Verification items for this drawing (mm, ordinates from the low corner). A direction names the side the tool comes from. Coordinates: 2 decimals unless noted, no trailing zeros. Order: outer loops, then holes, each group sorted by start corner. A loop starts at its lowest first (then second) coordinate and runs counter-clockwise, first axis right, second up.
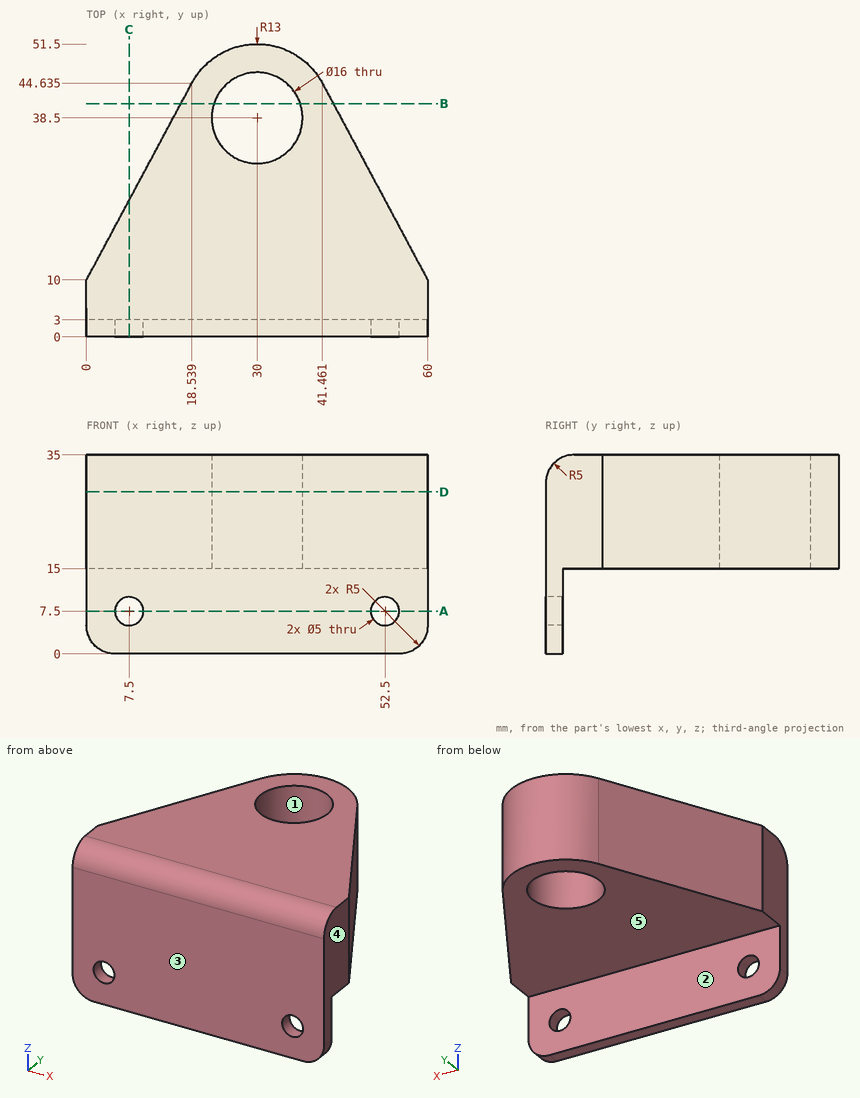
(1) Cross-section at A-A (z = 7.5). Enter the section's corners in (x, y), and give its area (3 significant figures).
Filled in:
outline: (0, 0) - (5, 0) - (5, 3) - (0, 3) - close; (10, 0) - (50, 0) - (50, 3) - (10, 3) - close; (55, 0) - (60, 0) - (60, 3) - (55, 3) - close
area: 150 mm2
(2) Cross-section at B-B (y = 41). Enter the section's corners in (x, z), and give its area (3 significant figures).
Filled in:
outline: (16.59, 15) - (22.4, 15) - (22.4, 35) - (16.59, 35) - close; (37.6, 15) - (43.41, 15) - (43.41, 35) - (37.6, 35) - close
area: 232 mm2
(3) Thickness scan on probe 1 along Y at (x, z) = (30, 22); probe 2 along X at (y, z) = (1, 7); probe 3 along Y at (x, z) = (57, 14). Record the ranges inside material, lowest first.
Filled in:
probe 1: y = 0 to 30.5, 46.5 to 51.5
probe 2: x = 0 to 5.05, 9.95 to 50.05, 54.95 to 60
probe 3: y = 0 to 3
(4) Cross-section at C-C (x = 7.5). Enter the section's corners in (y, z), and give its area (3 significant figures).
Filled in:
outline: (0, 0) - (3, 0) - (3, 5) - (0, 5) - close; (0, 10) - (3, 10) - (3, 15) - (24.01, 15) - (24.01, 35) - (5, 35) arc R5 ccw to (0, 30) - close
area: 505 mm2
(5) Release check for a two-part mould opening along Y. For the marked faces 1, 2 and 3 record: +Y half, -Y half, draft (parallel to the pull), parting line (faces both ways), or undercut.
Filled in:
face 1: undercut
face 2: +Y half
face 3: -Y half
(6) Tool access check on the marked faces 4 and 5. Record the directions out of +Z, -Z, +X, -X, +Y, -Y that give a thin tool (end or side, any length) a straight path to the whole face; none if there is none.
Filled in:
face 4: +Z, -Z, +X, +Y, -Y
face 5: -Z, +X, -X, +Y
(7) Go/stop test with flat-tipped pins: P1, Ø1, axis at x = 6, y = 12.5, coming from the -Z side; P2, Ø6, axis at x = 43.5, z = 28.5, coming from the +Y side (1 decimal); P3, Ø4.5, axis at x = 35, z = 4, coming from the +Y side. Record where each tip stops, or that it passes through.
Filled in:
P1: stops at z = 15
P2: stops at y = 46.2
P3: stops at y = 3
(8) Cross-section at D-D (z = 28.5). Enter the section's corners in (x, y) (1 decimal).
Filled in:
outline: (0, 0) - (60, 0) - (60, 10) - (41.5, 44.6) arc R13 ccw to (18.5, 44.6) - (0, 10) - close; hole circle Ø16 at (30, 38.5)
